from build123d import *
from build123d.topology import SkipClean

# Parameters (mm, degrees)
LEFT_ARM_DEPTH                = 12.5
SKETCH2_R                     = 37.5
LEFT_BOSS_DEPTH               = 37.5
LEFT_HEX_DEPTH                = 266.753645
LEFT_HEX_DEPTH_BACK           = 266.753645
SKETCH3_R                     = 50
CENTRE_BOSS_DEPTH             = 35
SKETCH5_W                     = 25
SKETCH5_H                     = 40
RIGHT_ARM_DEPTH               = 200
SKETCH7_R                     = 50
RIGHT_BOSS_DEPTH              = 37.5
SKETCH8_R                     = 34
RIGHT_BOSS_HOLE_DEPTH         = 461.862196
SKETCH9_R                     = 40
CENTRE_HOLE_DEPTH             = 461.461957
SKETCH10_R                    = 27.5
CENTRE_BLOB_DEPTH             = 35
CENTRE_BEAM_REACH             = 268.273
SKETCH11_W                    = 10
SKETCH11_H                    = 30
CENTRE_BEAM_DIRECTION_2_REACH = 268.273
SKETCH12_R                    = 20
CUT_EXTRUDE4_DEPTH            = 5
M6X1_0_TAPPED_HOLE1_D         = 5
CIRPATTERN1_COUNT             = 6
CUT_OUT_DEPTH                 = 10
FILLET1_R                     = 10
FILLET1_OF_MIRROR2_R          = 10
KEYWAY_DEPTH                  = 457.26222


with BuildPart() as part:
    # Sketch1 → LEFT_ARM (new, symmetric)
    with BuildSketch(Plane.XY):
        with BuildLine():
            Line((-2.34375, 37.426686), (196.875, 49.902248))
            ThreePointArc((196.875, 49.902248), (250, 0), (196.875, -49.902248))
            Line((196.875, -49.902248), (-2.34375, -37.426686))
            ThreePointArc((-2.34375, -37.426686), (-37.5, 0), (-2.34375, 37.426686))
        make_face()
    extrude(amount=LEFT_ARM_DEPTH, both=True)

    # Sketch2 → LEFT_Boss (add, symmetric)
    with SkipClean():  # the faces are left unmerged after this step: merging them gives an invalid solid
        with BuildSketch(Plane.XY):
            Circle(SKETCH2_R)
        extrude(amount=LEFT_BOSS_DEPTH, both=True)

    # Sketch4 → LEFT_Hex (cut, two sides: drawn at the far end of the back side and taken through both)
    with SkipClean():  # the faces are left unmerged after this step: merging them gives an invalid solid
        with BuildSketch(Plane.XY.offset(37.5).offset(-LEFT_HEX_DEPTH_BACK)):
            Polygon((23.094011, 0), (11.547005, 20), (-11.547005, 20), (-23.094011, 0), (-11.547005, -20), (11.547005, -20), align=None)
        extrude(amount=LEFT_HEX_DEPTH + LEFT_HEX_DEPTH_BACK, mode=Mode.SUBTRACT)

    # Sketch3 → CENTRE_Boss (add, symmetric)
    with SkipClean():  # the faces are left unmerged after this step: merging them gives an invalid solid
        with BuildSketch(Plane.XY):
            with Locations((200, 0)):
                Circle(SKETCH3_R)
        extrude(amount=CENTRE_BOSS_DEPTH, both=True)

    # Sketch5 → RIGHT_ARM (add)
    with SkipClean():  # the faces are left unmerged after this step: merging them gives an invalid solid
        with BuildSketch(Plane(origin=(186.60254, 50, 0), x_dir=(0, 0, -1), z_dir=(0.9659258262890681, 0.25881904510252135, 0))):
            with Locations((0, -51.763809)):
                Rectangle(SKETCH5_W, SKETCH5_H)
        extrude(amount=RIGHT_ARM_DEPTH)

    # Sketch7 → RIGHT_Boss (add, symmetric)
    with SkipClean():  # the faces are left unmerged after this step: merging them gives an invalid solid
        with BuildSketch(Plane.XY):
            with Locations((393.185165, 51.763809)):
                Circle(SKETCH7_R)
        extrude(amount=RIGHT_BOSS_DEPTH, both=True)

    # Sketch8 → RIGHT_Boss_Hole (cut, through all)
    with SkipClean():  # the faces are left unmerged after this step: merging them gives an invalid solid
        with BuildSketch(Plane.XY.offset(37.5)):
            with Locations((393.185165, 51.763809)):
                Circle(SKETCH8_R)
        extrude(amount=-RIGHT_BOSS_HOLE_DEPTH, mode=Mode.SUBTRACT)

    # Sketch9 → CENTRE_Hole (cut, through all)
    with SkipClean():  # the faces are left unmerged after this step: merging them gives an invalid solid
        with BuildSketch(Plane.XY.offset(35)):
            with Locations((200, 0)):
                Circle(SKETCH9_R)
        extrude(amount=-CENTRE_HOLE_DEPTH, mode=Mode.SUBTRACT)

    # Sketch10 → CENTRE_Blob (add, symmetric)
    with SkipClean():  # the faces are left unmerged after this step: merging them gives an invalid solid
        with BuildSketch(Plane.XY):
            with Locations((224.148146, 6.470476)):
                Circle(SKETCH10_R)
        extrude(amount=CENTRE_BLOB_DEPTH, both=True)

    # Sketch11 → CENTRE_Beam (add, up to next)
    with BuildSketch(Plane(origin=(200, 0, 0), x_dir=(0, 0, -1), z_dir=(1, 0, 0)), mode=Mode.PRIVATE) as centre_beam_sk1:
        Rectangle(SKETCH11_W, SKETCH11_H)
    centre_beam_tool1 = extrude(centre_beam_sk1.sketch, amount=CENTRE_BEAM_REACH, mode=Mode.PRIVATE) - part.part
    add(centre_beam_tool1.solids().sort_by_distance((200, 0, 0))[0])

    # Sketch11 → CENTRE_Beam direction 2 (add, up to next)
    with BuildSketch(Plane(origin=(200, 0, 0), x_dir=(0, 0, -1), z_dir=(1, 0, 0)), mode=Mode.PRIVATE) as centre_beam_direction_2_sk1:
        Rectangle(SKETCH11_W, SKETCH11_H)
    centre_beam_direction_2_tool1 = extrude(centre_beam_direction_2_sk1.sketch, amount=-CENTRE_BEAM_DIRECTION_2_REACH, mode=Mode.PRIVATE) - part.part
    add(centre_beam_direction_2_tool1.solids().sort_by_distance((200, 0, 0))[0])

    # Sketch12 → Cut-Extrude4 (cut)
    with SkipClean():  # the faces are left unmerged after this step: merging them gives an invalid solid
        with BuildSketch(Plane.XY.offset(35)):
            with Locations((224.148146, 6.470476)):
                Circle(SKETCH12_R)
        cut_extrude4 = extrude(amount=-CUT_EXTRUDE4_DEPTH, mode=Mode.SUBTRACT)

    # M6x1.0 Tapped Hole1 (through all)
    with Locations(Plane.XY.offset(30)):
        with Locations((209.659258, 2.58819)):
            m6x1_0_tapped_hole1 = Hole(M6X1_0_TAPPED_HOLE1_D / 2)

    # CirPattern1: M6x1.0 Tapped Hole1 ×6 about axis
    with SkipClean():  # the faces are left unmerged after this step: merging them gives an invalid solid
        cirpattern1_axis = Axis((224.148146, 6.470476, 0), (0, 0, 1))
        for i in range(1, CIRPATTERN1_COUNT):
            add(m6x1_0_tapped_hole1.rotate(cirpattern1_axis, i * 360 / CIRPATTERN1_COUNT), mode=Mode.SUBTRACT)

    # Mirror1: Cut-Extrude4 across plane
    with SkipClean():  # the faces are left unmerged after this step: merging them gives an invalid solid
        add(cut_extrude4.mirror(Plane.XY), mode=Mode.SUBTRACT)

    # Sketch15 → Cut_OUT (cut)
    with SkipClean():  # the faces are left unmerged after this step: merging them gives an invalid solid
        with BuildSketch(Plane.XY.offset(12.5)):
            with BuildLine():
                Line((152.866072, 37.126714), (36.935365, 29.866851))
                ThreePointArc((36.935365, 29.866851), (47.5, 0), (36.935365, -29.866851))
                Line((36.935365, -29.866851), (152.866072, -37.126714))
                ThreePointArc((152.866072, -37.126714), (140, 0), (152.866072, 37.126714))
            make_face()
        cut_out = extrude(amount=-CUT_OUT_DEPTH, mode=Mode.SUBTRACT)

    # Fillet1
    fillet1_edges = [part.edges().sort_by_distance(p)[0] for p in [
        (36.935365, -29.866851, 7.5),
        (36.935365, 29.866851, 7.5),
        (152.866072, 37.126714, 7.5),
        (152.866072, -37.126714, 7.5),
    ]]
    fillet(fillet1_edges, radius=FILLET1_R)

    # Mirror2: Cut_OUT across plane
    with SkipClean():  # the faces are left unmerged after this step: merging them gives an invalid solid
        add(cut_out.mirror(Plane.XY), mode=Mode.SUBTRACT)

    # Fillet1 of Mirror2
    fillet1_of_mirror2_edges = [part.edges().sort_by_distance(p)[0] for p in [
        (36.935365, -29.866851, -7.5),
        (36.935365, 29.866851, -7.5),
        (152.866072, 37.126714, -7.5),
        (152.866072, -37.126714, -7.5),
    ]]
    fillet(fillet1_of_mirror2_edges, radius=FILLET1_OF_MIRROR2_R)

    # Sketch16 → KEYWAY (cut, symmetric)
    with SkipClean():  # the faces are left unmerged after this step: merging them gives an invalid solid
        with BuildSketch(Plane.XY):
            Polygon((395.773356, 42.104551), (390.596975, 61.423067), (353.505423, 51.484416), (358.681804, 32.165899), align=None)
        keyway = extrude(amount=KEYWAY_DEPTH, both=True, mode=Mode.SUBTRACT)

    # Mirror3: KEYWAY across plane
    with SkipClean():  # the faces are left unmerged after this step: merging them gives an invalid solid
        add(keyway.mirror(Plane(origin=(379.787706, 101.763809, 0), x_dir=(0, 0, 1), z_dir=(0.9659258262890681, 0.25881904510252135, 0))), mode=Mode.SUBTRACT)


solid = part.part
Read the model definition and answer for the solid it produces. Units are mm, in the model's axes. A direction names the side the tool comes from. Coordinates: 2 decimals unless noted, no trailing zeros. Loops run counter-clockwise (first coordinate to the right, second up) from the corner with the lowest first, then second, coordinate; pieces in that order, holes last.
Q1. The part is cut by section B-B on x = 84. Write down the section's boundary in (y, z), and give its area (3 significant figures).
Q2. Consider probe 1 along X at (y, z) = (6, 24.5); probe 2 along X at (y, z) = (-8, 29); probe 3 along Y at (x, z) = (227, 12). Determine where each line is inside the solid, lowest interval first.
Q3. The mould has two halves that part along Y. Classify faces 4 (the face through (296, 25, 12.5)), 5 (the face through (95.871, 43.577, 0.175)), 6 (the face through (93.092, -33.384, 7.57)), 7 (the face through (401.4, 18.77, 0.52)): +Y half, -Y half, draft (parallel to the pull), parting line (faces both ways), or undercut.
Q4. The part is cut by section C-C on x = 306. Write down the section's boundary in (y, z).
Q5. Which of the six approach directions +Z, -Z, +X, -X, +Y, -Y give full straight-line access (tool end or side, diameter ignored) to faces 1 (the face through (17.24, -10.14, -0.53)), 2 (the face through (47.5, 0.2, -7.6)), 3 (the face through (83, 34, 12.5))?
Q6. The part is cut by section A-A on z = -19. Give the number of separate pieces and of enclosed holes in the cut face, and give its area (3 significant figures).
Q7. Each of these flat-tipped pins is pushed along its axis until it touches: pin 1 Ø4 at (x, y) = (72, 20.5) entering from +Z; pin 2 Ø3 at (y, z) = (-33, 4) entering from -X; pin 3 Ø10 at (x, z) = (200, -9) entering from +Y. Where does it stop, or does it pass through?
Results below:
1. outline: (-42.83, -12.5) - (-32.81, -12.5) - (-32.81, -2.5) - (32.81, -2.5) - (32.81, -12.5) - (42.83, -12.5) - (42.83, 12.5) - (32.81, 12.5) - (32.81, 2.5) - (-32.81, 2.5) - (-32.81, 12.5) - (-42.83, 12.5) - close
1. area: 829 mm2
2. probe 1: x = -37.02 to -19.63, 19.63 to 37.02, 150.36 to 160.45, 196.65 to 251.64, 373.04 to 413.33
2. probe 2: x = -36.64 to -18.48, 18.48 to 36.64, 150.64 to 160.81, 200.76 to 217.77, 222.77 to 249.36
2. probe 3: y = -42.08 to -29.51, -20.88 to 18.68, 23.24 to 42.08
3. face 4: draft
3. face 5: +Y half
3. face 6: undercut
3. face 7: undercut
4. outline: (7.7, -12.5) - (49.11, -12.5) - (49.11, 12.5) - (7.7, 12.5) - close
5. face 1: +Z, -Z
5. face 2: -Z
5. face 3: +Z
6. separate pieces: 3
6. enclosed holes: 9
6. area: 11,600 mm2
7. pin 1: stops at z = 2.5
7. pin 2: stops at x = -20.35
7. pin 3: stops at y = 50
